```python
from build123d import *

# Parameters (mm, degrees)
F0_W     = 76.2
F0_H     = 50.8
F1_DEPTH = 12.7
F2_R     = 12.7
F3_DEPTH = 25.4
F4_W     = 1.281619072
F4_H     = 0.3408930868
F4_H_2   = 4.7445660457
F5_DEPTH = 50.8508


with BuildPart() as f1:
    # F0 (on Top) → F1 (new body)
    with BuildSketch(Plane.XY):
        Rectangle(F0_W, F0_H)
    extrude(amount=F1_DEPTH)

    # F2 (on face) → F3 (cut)
    with BuildSketch(Plane.XY.offset(12.7)):
        Circle(F2_R)
    extrude(amount=-F3_DEPTH, mode=Mode.SUBTRACT)

    # F4 (on face) → F5 (cut)
    with BuildSketch(Plane.XZ.offset(25.4)):
        with Locations((-34.9193550646, 12.5295534566)):
            Rectangle(F4_W, F4_H)
        with Locations((-34.9193550646, 9.9868238904)):
            Rectangle(F4_W, F4_H_2)
    extrude(amount=-F5_DEPTH, mode=Mode.SUBTRACT)


solid = f1.part
```
Could you check a few things on this model? Use its own coordinates, in mm. A direction names the side the tool comes from. Round coordinates to 2 decimals unless told otherwise and drop trailing zeros. Loops run counter-clockwise (first coordinate to the right, second up) from the corner with the lowest first, then second, coordinate; pieces in that order, holes last. Notation, with made-up numbers: (51, -23.75) - (59, -23.75) arc R18 cw to (59, -10.75) - close; hole circle Ø4 at (-9, 10.25). An arc over 180 degrees is marked (long way). Answer as CSV lines item,"result".
1. I want a section at A-A on z = 11.5. List the corners of the cut face in (x, y) for me.
Filled in:
outline,"(-38.1, -25.4) - (-35.56, -25.4) - (-35.56, 25.4) - (-38.1, 25.4) - close; (-34.28, -25.4) - (38.1, -25.4) - (38.1, 25.4) - (-34.28, 25.4) - close; hole circle Ø25.4 at (0, 0)"
2. We'd pull the mould along X, two halves only. Please class faces 1 (the face through (-1, 25.4, 6)), 2 (the face through (-38.1, 0, 6)), 3 (the face through (-34.279, 0, 10)): +X half, -X half, draft (parallel to the pull), parting line (faces both ways), or undercut.
Filled in:
face 1,"draft"
face 2,"-X half"
face 3,"undercut"
3. Please list where these lines run through material, in increasing order: line 1 along X through (y, z) = (10, 11.75); line 2 along Y through (x, z) = (0, 9.25); line 3 along X through (y, z) = (21, 11.5). Write a range as [from, to].
Filled in:
line 1,"x = [-38.1, -35.56], [-34.28, -7.83], [7.83, 38.1]"
line 2,"y = [-25.4, -12.7], [12.7, 25.4]"
line 3,"x = [-38.1, -35.56], [-34.28, 38.1]"
4. I want a section at B-B on x = 0. List the corners of the cut face in (y, z) for me, then the cut area to 3 significant figures.
Filled in:
outline,"(-25.4, 0) - (-12.7, 0) - (-12.7, 12.7) - (-25.4, 12.7) - close; (12.7, 0) - (25.4, 0) - (25.4, 12.7) - (12.7, 12.7) - close"
area,"323 mm^2"
5. I want a section at D-D on z = 4. List the corners of the cut face in (x, y) for me, then the cut area to 3 significant figures.
Filled in:
outline,"(-38.1, -25.4) - (38.1, -25.4) - (38.1, 25.4) - (-38.1, 25.4) - close; hole circle Ø25.4 at (0, 0)"
area,"3,360 mm^2"
6. I want a section at C-C on y = 8. List the corners of the cut face in (x, z) for me, then the cut area to 3 significant figures.
Filled in:
outline,"(-38.1, 0) - (-9.86, 0) - (-9.86, 12.7) - (-34.28, 12.7) - (-34.28, 7.61) - (-35.56, 7.61) - (-35.56, 12.7) - (-38.1, 12.7) - close; (9.86, 0) - (38.1, 0) - (38.1, 12.7) - (9.86, 12.7) - close"
area,"711 mm^2"
7. On a 3-axis mill with a long thin cutter (end or side, diameter ignored), from which of +Z, -Z, +X, -X, +Y, -Y can I reach the whole of each face in a straight line? I mean faces 4 (the face through (-35.56, 0, 10)), 5 (the face through (8, 12, 0)). Say none if no direction works.
Filled in:
face 4,"+Z, +Y, -Y"
face 5,"-Z, +X, -X, +Y, -Y"
